from build123d import *

# Parameters (mm, degrees)
F0_W     = 152
F0_H     = 152
F0_R     = 7
F1_DEPTH = 5
F3_DEPTH = 88.9
F4_R     = 5
F5_R     = 1
F7_D     = 14
F9_D     = 14


# Not quite as in the source:
# - a feature names something its author has since deleted; it is built from what else it names


with BuildPart() as f1:
    # F0 (on Top) → F1 (new body)
    with BuildSketch(Plane.XY):
        Rectangle(F0_W, F0_H)
        with Locations((-54, -54)):
            Circle(F0_R, mode=Mode.SUBTRACT)
        with Locations((54, -54)):
            Circle(F0_R, mode=Mode.SUBTRACT)
        with Locations((-54, 54)):
            Circle(F0_R, mode=Mode.SUBTRACT)
        with Locations((54, 54)):
            Circle(F0_R, mode=Mode.SUBTRACT)
    extrude(amount=-F1_DEPTH)

    # F2 (on face) → F3 (join)
    with BuildSketch(Plane.XY):
        Polygon((-21, 20.65), (-23.5, 20.65), (-23.5, -23.15), (23.5, -23.15), (23.5, 20.65), (21, 20.65), (21, -20.65), (-21, -20.65), align=None)
    extrude(amount=F3_DEPTH)

    # F4
    f4_edges = [f1.edges().sort_by_distance(p)[0] for p in [
        (23.5, -23.15, 44.45),
        (-23.5, -23.15, 44.45),
    ]]
    fillet(f4_edges, radius=F4_R)

    # F5
    f5_edges = [f1.edges().sort_by_distance(p)[0] for p in [
        (21, -20.65, 44.45),
        (-21, -20.65, 44.45),
    ]]
    fillet(f5_edges, radius=F5_R)

    # F7 (through all)
    with Locations(Plane.YZ.offset(23.5)):
        with Locations((0, 67.9), (0, 19.9)):
            Hole(F7_D / 2)

    # F9 (through all)
    with Locations(Plane.XZ.offset(23.15)):
        with Locations((0, 67.9), (0, 19.9)):
            Hole(F9_D / 2)


solid = f1.part
Could you check a few things on this model? Use its own coordinates, in mm. A direction names the side the tool comes from. Give positions to 0.01 mm unless a question says otherwise; leave off trailing zeros. Write each loop counter-clockwise with the first axis right and the second up, starting at its lowest first coordinate (ties: lowest second). Pieces come first, ordered by that corner, then holes. Notation, with made-up numbers: (33, 53) -> (55, 53) arc R11 cw to (55, 60) -> close; hole circle Ø3 at (21.25, 47.25). An arc over 180 degrees is marked (long way). Answer as CSV lines item,"result". Start each with the question number.
(1) If we section it at D-D, the plane y = 9.5: Write out the boundary of the cut face in (x, z), and give its area (3 significant figures).
(2) If we mould it in two halves opening along Z, with no side actions, what happens to faces 1 (the face through (22.23, 0.91, 26.84)), 2 (the face through (-1, 1, 0)), 3 (the face through (0, -23.15, 44))? For each: +Z half, -Z half, draft (parallel to the pull), parting line (faces both ways), or undercut.
(3) If we section it at A-A, the plane x = -54: Write out the boundary of the cut face in (y, z).
(4) Please list where these lines run through material, in increasing order: line 1 (Y direction, x = -54, z = -1); line 2 (Z direction, x = 0, y = -21); line 3 (X direction, y = -7.5, z = 77).
(5) I'm going to push flat-ended pins straight in: pin 1 Ø10 at (y, z) = (-16.5, 30) entering from +X; pin 2 Ø1 at (x, y) = (21, 54.5) entering from +Z; pin 3 Ø2 at (x, z) = (-22, 51) entering from +Y. Where does each tip first touch, or does it pass through?
(6) If we section it at B-B, the plane z = 19.9: Write out the boundary of the cut face in (x, y), and give its area (3 significant figures).
(7) Which directions (+Z, -Z, +X, -X, +Y, -Y) give clear straight access to the entire face, cutting with the end or side of a thin tool? Please do faces 4 (the face through (23.5, 1, 44)), 5 (the face through (-21, 0, 44)), 6 (the face through (-23.5, 2, 44)), 7 (the face through (22, -21.72, 45.07)).
Answer list:
1,outline,"(-76, -5) -> (76, -5) -> (76, 0) -> (23.5, 0) -> (23.5, 88.9) -> (21, 88.9) -> (21, 0) -> (-21, 0) -> (-21, 88.9) -> (-23.5, 88.9) -> (-23.5, 0) -> (-76, 0) -> close"
1,area,"1,200 mm^2"
2,face 1,"undercut"
2,face 2,"+Z half"
2,face 3,"draft"
3,outline,"(-76, -5) -> (-61, -5) -> (-61, 0) -> (-76, 0) -> close; (-47, -5) -> (47, -5) -> (47, 0) -> (-47, 0) -> close; (61, -5) -> (76, -5) -> (76, 0) -> (61, 0) -> close"
4,line 1,"-76 to -61, -47 to 47, 61 to 76"
4,line 2,"-5 to 12.9, 26.9 to 60.9, 74.9 to 88.9"
4,line 3,"-23.5 to -21, 21 to 23.5"
5,pin 1,"x = 23.5"
5,pin 2,"z = 0"
5,pin 3,"y = 20.65"
6,outline,"(-23.5, -18.15) arc R5 ccw to (-18.5, -23.15) -> (-7, -23.15) -> (-7, -20.65) -> (-20, -20.65) arc R1 cw to (-21, -19.65) -> (-21, -7) -> (-23.5, -7) -> close; (-23.5, 7) -> (-21, 7) -> (-21, 20.65) -> (-23.5, 20.65) -> close; (7, -23.15) -> (18.5, -23.15) arc R5 ccw to (23.5, -18.15) -> (23.5, -7) -> (21, -7) -> (21, -19.65) arc R1 cw to (20, -20.65) -> (7, -20.65) -> close; (21, 7) -> (23.5, 7) -> (23.5, 20.65) -> (21, 20.65) -> close"
6,area,"209 mm^2"
7,face 4,"+Z, +X, +Y, -Y"
7,face 5,"+Z, +Y"
7,face 6,"+Z, -X, +Y, -Y"
7,face 7,"+Z, +X, -Y"
